For this review, use the dimensioned drawing (mm, ordinates from the lowest corner) and the shaded views. A direction names the side the tool comes from. Round coordinates to 2 decimals unless told otherwise and drop trailing zeros. Loops run counter-clockwise (first coordinate to the right, second up) from the corner with the lowest first, then second, coordinate; pieces in that order, holes last. Notation, with made-up numbers: (62, 37) -> (107, 37) arc R10 cw to (107, 51) -> close; hole circle Ø10 at (63.25, -11). An arc over 180 degrees is marked (long way). Write each question's results on one line, items separated by ' | '. Start each with the question number.
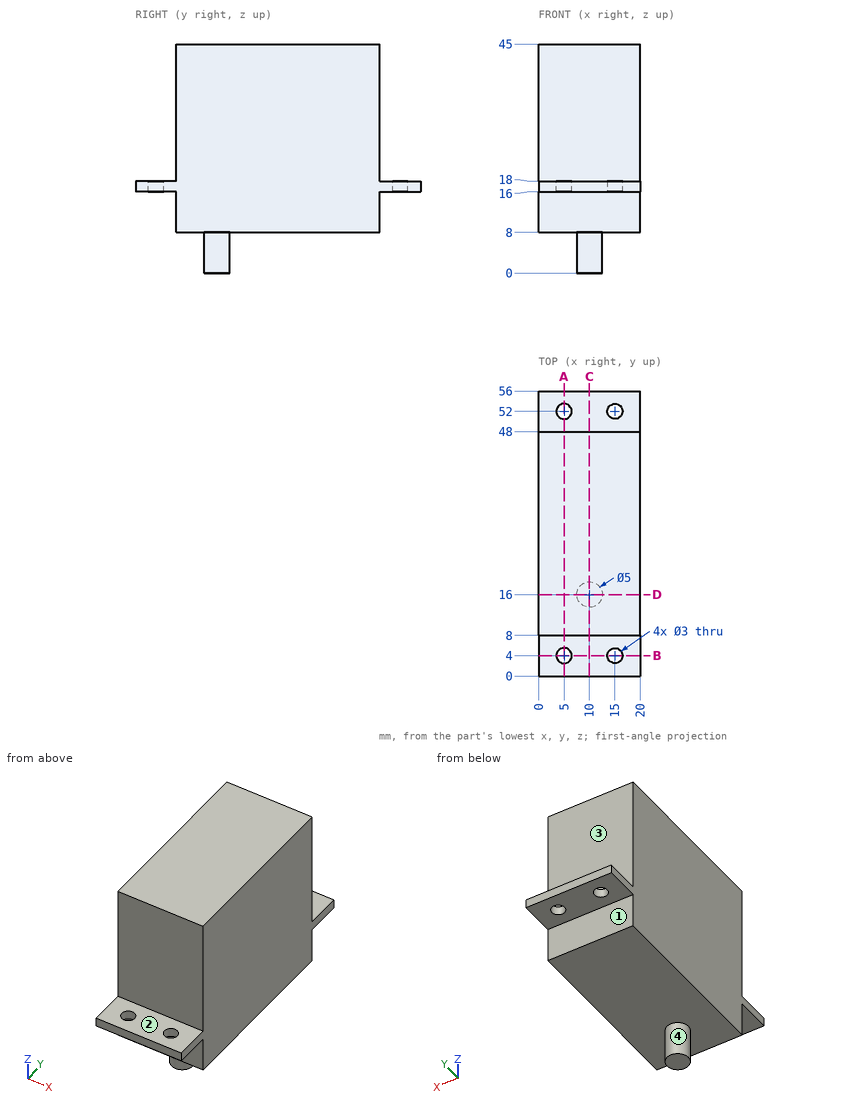
1) For the marked faces 1, 2, 3 and 4, list the 3-axis set-ups (+Z, -Z, +X, -X, +Y, -Y) from which the entire face can be reached by the end or side of a thin tool; tool diameter is ignored.
2) Take a section at D-D (y = 16). Write out the cut boundary in (x, z).
3) Take a section at C-C (x = 10). Write out the cut boundary in (y, z).
4) Take a section at B-B (y = 4). Write out the cut boundary in (x, z), plus the area to 3 significant figures.
5) Take a section at A-A (x = 5). Write out the cut boundary in (y, z).
6) To check wall thickness, follow line 1 (Y direction, x = 15, z = 16.5); line 2 (Y direction, x = 10.25, z = 35); line 3 (Z direction, x = 7.75, y = 20). State the ranges of each line that lie inside material, in increasing order. Write a range as from..to.
7) Insertion check: pin 1 (2.5 mm diameter, centred on x = 5, y = 52, fed in from +Z); pin 2 (6.5 mm diameter, centred on x = 12, y = 52, fed in from +Z); pin 3 (2.5 mm diameter, centred on x = 14, z = 12.5, fed in from +Y); pin 4 (2.5 mm diameter, centred on x = 9, y = 4.5, fed in from -Z). Each pin has a flat end and moves straight along its axis. Give the tip position at first contact, or say it passes through.
Geometry check:
1) face 1: -Z, +X, -X, +Y | face 2: +Z, +X, -X, -Y | face 3: +Z, +X, -X, +Y | face 4: -Z
2) outline: (0, 8) -> (7.5, 8) -> (7.5, 0) -> (12.5, 0) -> (12.5, 8) -> (20, 8) -> (20, 45) -> (0, 45) -> close
3) outline: (0, 16) -> (8, 16) -> (8, 8) -> (13.5, 8) -> (13.5, 0) -> (18.5, 0) -> (18.5, 8) -> (48, 8) -> (48, 16) -> (56, 16) -> (56, 18) -> (48, 18) -> (48, 45) -> (8, 45) -> (8, 18) -> (0, 18) -> close
4) outline: (0, 16) -> (3.5, 16) -> (3.5, 18) -> (0, 18) -> close; (6.5, 16) -> (13.5, 16) -> (13.5, 18) -> (6.5, 18) -> close; (16.5, 16) -> (20, 16) -> (20, 18) -> (16.5, 18) -> close | area: 28.0 mm^2
5) outline: (0, 16) -> (2.5, 16) -> (2.5, 18) -> (0, 18) -> close; (5.5, 16) -> (8, 16) -> (8, 8) -> (48, 8) -> (48, 16) -> (50.5, 16) -> (50.5, 18) -> (48, 18) -> (48, 45) -> (8, 45) -> (8, 18) -> (5.5, 18) -> close; (53.5, 16) -> (56, 16) -> (56, 18) -> (53.5, 18) -> close
6) line 1: y = 0..2.5, 5.5..50.5, 53.5..56 | line 2: y = 8..48 | line 3: z = 8..45
7) pin 1: passes through | pin 2: stops at z = 18 | pin 3: stops at y = 48 | pin 4: stops at z = 16
